from build123d import *

# Parameters (mm, degrees)
F2_SIZE  = 0.25
F3_W     = 15
F3_H     = 1.2
F4_DEPTH = 8
F5_R     = 1
F6_DEPTH = 12.5


with BuildPart() as f1:
    # F0 (on Front) → F1 (revolve)
    with BuildSketch(Plane.XZ):
        Polygon((0, 7), (0, 0), (29, 0), (29, 2), (26.113249, 7), (22.5, 7), (22, 6.133975), (21.5, 7), (17.5, 7), (17, 6.133975), (16.5, 7), (12.5, 7), (12, 6.133975), (11.5, 7), align=None)
    revolve(axis=Axis((14.5, 0, 0), (-1, 0, 0)))

    # F2
    f2_edges = [f1.edges().sort_by_distance(p)[0] for p in [
        (0, 0, -7),
    ]]
    chamfer(f2_edges, length=F2_SIZE)

    # F3 (on Right) → F4 (cut)
    with BuildSketch(Plane.YZ):
        Rectangle(F3_W, F3_H)
    extrude(amount=F4_DEPTH, mode=Mode.SUBTRACT)

    # F5 (on Top) → F6 (cut, symmetric)
    with BuildSketch(Plane.XY):
        with Locations((4, 0)):
            Circle(F5_R)
    extrude(amount=F6_DEPTH, both=True, mode=Mode.SUBTRACT)


solid = f1.part
Source: CAD feature listing. Evaluate the final solid. Frame: model axes, mm. A direction names the side the tool comes from. Coordinates: 2 decimals unless noted, no trailing zeros. Order: outer loops, then holes, each group sorted by start corner. A loop starts at its lowest first (then second) coordinate and runs counter-clockwise, first axis right, second up.
Item 1: Cut plane D-D (y = 0). Count the separate pieces of the cut face and the enclosed holes in it, plus the area to 3 significant figures.
Output values:
separate pieces: 3
enclosed holes: 0
area: 354 mm2
Item 2: Pull-direction query (Y, two-part tool) for faces 1 (the face through (3.9, 1.5, 0.6)), 2 (the face through (0.13, 0.14, -6.88)), 3 (the face through (3, 0, -4)); classes: pulls with the +Y half, pulls with the -Y half, needs draft (parallel to the pull), parting line crosses it, or undercut.
Output values:
face 1: needs draft
face 2: parting line crosses it
face 3: undercut
Item 3: First-contact query: P1, Ø1.5, axis at x = 10, z = 1, coming from the -Y side; P2, Ø0.6, axis at y = 0, z = 0, coming from the -X side; P3, Ø1.6, axis at x = 4, y = 0, coming from the -Z side; P4, Ø3, axis at x = 4.5, z = 4.5, coming from the +Y side. Flat tips, straight axial feed; report the tip coordinate or a pass-through.
Output values:
P1: stops at y = -7
P2: stops at x = 8
P3: passes through
P4: stops at y = 6.32
Item 4: Cut plane A-A (x = 4). Return loops of the section in (y, z), plus the area to 3 significant figures.
Output values:
outline: (-6.97, -0.6) arc R7 ccw to (-1, -6.93) - (-1, -0.6) - close; (-6.97, 0.6) - (-1, 0.6) - (-1, 6.93) arc R7 ccw to start; (1, -6.93) arc R7 ccw to (6.97, -0.6) - (1, -0.6) - close; (1, 0.6) - (6.97, 0.6) arc R7 ccw to (1, 6.93) - close
area: 112 mm2
Item 5: Set-up query: faces 4 (the face through (5.796, -2.681, 6.466)), 5 (the face through (8, 0, 0)). Return all of +Z, -Z, +X, -X, +Y, -Y with unobstructed straight access to the full face (end or side cutting, diameter ignored); none if empty.
Output values:
face 4: +X, -X
face 5: -X, +Y, -Y
Item 6: Cut plane C-C (z = 0). Return loops of the section in (x, y).
Output values:
outline: (8, -7) - (11.5, -7) - (12, -6.13) - (12.5, -7) - (16.5, -7) - (17, -6.13) - (17.5, -7) - (21.5, -7) - (22, -6.13) - (22.5, -7) - (26.11, -7) - (29, -2) - (29, 2) - (26.11, 7) - (22.5, 7) - (22, 6.13) - (21.5, 7) - (17.5, 7) - (17, 6.13) - (16.5, 7) - (12.5, 7) - (12, 6.13) - (11.5, 7) - (8, 7) - close
Item 7: Material intervals for line 1 (Z direction, x = 22.75, y = -0.25); line 2 (X direction, y = 0, z = -2); line 3 (Z direction, x = 3.25, y = 4.5), sorted ascending.
Output values:
line 1: z = -7 to 7
line 2: x = 0 to 3, 5 to 29
line 3: z = -5.36 to -0.6, 0.6 to 5.36
